Autodesk Inventor part; units mm, degrees
ref_plane "YZ Plane" through (0, 0, 0) normal (1, 0, 0) x (0, 1, 0)
ref_plane "XZ Plane" through (0, 0, 0) normal (0, 1, 0) x (-1, 0, 0)
ref_plane "XY Plane" through (0, 0, 0) normal (0, 0, 1) x (1, 0, 0)
sketch "Boceto1" plane through (0, 0, 0) normal (0, 1, 0) x (-1, 0, 0)
  line L0 (-40, -40) -> (40, -40)
  line L1 (40, -40) -> (40, 40)
  line L2 (40, 40) -> (-40, 40)
  line L3 (-40, 40) -> (-40, -40)
  line L4 (-40, -40) -> (40, 40) construction
  line L5 (40, -40) -> (-40, 40) construction
  point P0 (0, 0)
  dimension "d0" = 80
  dimension "d1" = 80
extrude "Extrusión1" add sketch "Boceto1" along normal blind 25
sketch "Boceto2" plane through (0, 25, 0) normal (0, 1, 0) x (1, 0, 0)
  line L0 (-40, -40) -> (40, -40)
  line L1 (40, -40) -> (40, 40)
  circle A0 centre (35.8, -35.8) radius 2.1
  line L2 (40, 40) -> (35.8, 40)
  line L3 (40, 40) -> (-40, 40)
  line L4 (35.8, 40) -> (40, 40)
  line L5 (-40, 40) -> (-40, -40)
  line L6 (-40, 40) -> (-35.8, 40)
  line L7 (-35.8, 40) -> (-35.8, 35.8)
  line L8 (-40, -40) -> (-35.8, -40)
  line L9 (-35.8, -40) -> (-35.8, -35.8)
  circle A1 centre (-35.8, -35.8) radius 2.1
  circle A2 centre (-35.8, 35.8) radius 2.1
  line L10 (35.8, 40) -> (35.8, 35.8)
  circle A3 centre (35.8, 35.8) radius 2.1
  point P0 (0, 0)
  dimension "d15" = 4.2
  dimension "d16" = 4.2
  dimension "d17" = 4.2
  dimension "d18" = 4.2
  dimension "d19" = 4.2
  dimension "d20" = 4.2
  dimension "d21" = 4.2
  dimension "d22" = 4.2
  dimension "d23" = 4.2
  dimension "d24" = 4.2
hole "Agujero1" at (35.8, 25, 35.8) at (35.8, 25, -35.8) at (-35.8, 25, -35.8) at (-35.8, 25, 35.8) direction (0, -1, 0) diameter 4.25 depth 30
properties part number "Ventilador"
Input: part model. Units: mm. Frame: model coordinates. Round coordinates to 2 decimals unless told otherwise and drop trailing zeros. Loops run counter-clockwise (first coordinate to the right, second up) from the corner with the lowest first, then second, coordinate; pieces in that order, holes last. Notation, with made-up numbers: (-38, -21.5) - (3, -21.5) arc R17 ccw to (3, -5.5) - close; hole circle Ø6 at (3.25, 89). An arc over 180 degrees is marked (long way). One line per item, written item: value. Start each with the question number.
(1) Draft query along X for faces 1 (the cylindrical face through (-37.907, 12.325, -36.077)), 2 (the flat face through (40, 12, 1)), 3 (the flat face through (1, 25, 1)). Return one class per face: +X half, -X half, draft (parallel to the pull), parting line (faces both ways), or undercut.
(2) Section B-B, the plane x = -35.8. Return loops of the section in (y, z) (3 decimals).
(3) Section A-A, the plane z = -35.8. Return loops of the section in (x, y) (3 decimals), plus the area to 3 significant figures.
(4) Ray query, line 1 (X direction, y = 5, z = 35.8) (3 decimals). Return the intervals inside material, ascending. Write a range as [from, to].
Results below:
1. face 1: undercut
1. face 2: +X half
1. face 3: draft
2. outline: (0, -40) - (25, -40) - (25, -37.925) - (0, -37.925) - close; (0, -33.675) - (25, -33.675) - (25, 33.675) - (0, 33.675) - close; (0, 37.925) - (25, 37.925) - (25, 40) - (0, 40) - close
3. outline: (-40, 0) - (-37.925, 0) - (-37.925, 25) - (-40, 25) - close; (-33.675, 0) - (33.675, 0) - (33.675, 25) - (-33.675, 25) - close; (37.925, 0) - (40, 0) - (40, 25) - (37.925, 25) - close
3. area: 1,790 mm^2
4. line 1: [-40, -37.925], [-33.675, 33.675], [37.925, 40]
